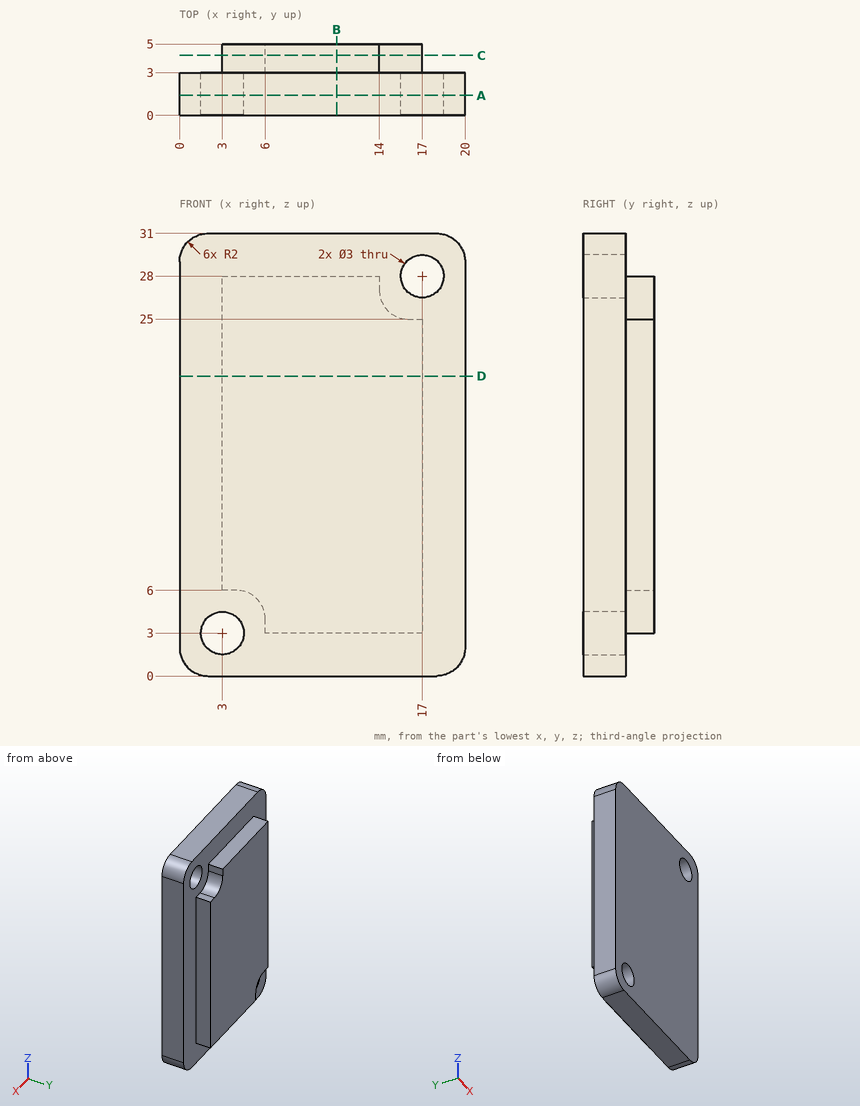
Print and shaded views of the part. All mm, measured from the part's lowest x, y and z. Round coordinates to 2 decimals unless told otherwise and drop trailing zeros. Order: outer loops, then holes, each group sorted by start corner. A loop starts at its lowest first (then second) coordinate and runs counter-clockwise, first axis right, second up.
Q1. Drop flat-ended pins along their axis: pin 1 (0.5 mm diameter, centred on x = 3.5, y = 3.5, fed in from -Z); pin 2 (3.5 mm diameter, centred on x = 17, z = 28, fed in from +Y); pin 3 (0.6 mm diameter, centred on x = 7.5, y = 4.5, fed in from +Z). Give the stop position or say it passes through.
Q2. Slice it at D-D (z = 21). Write the cut outline in (x, y), and give its area (3 significant figures).
Q3. Slice it at A-A (y = 1.4). Write the cut outline in (x, z).
Q4. Wall check: L1, parallel to X at y = 0.85, z = 28; L2, parallel to X at y = 1.3, z = 3; L3, parallel to Y at x = 1.75, z = 13.5. Give the ranges that are in metal, low to high.
Q5. Slice it at C-C (y = 4.2). Write the cut outline in (x, z).
Q6. Slice it at B-B (x = 11). Write the cut outline in (y, z), and give its area (3 significant figures).
Results below:
1. pin 1: stops at z = 6
1. pin 2: stops at y = 3
1. pin 3: stops at z = 28
2. outline: (0, 0) - (20, 0) - (20, 3) - (17, 3) - (17, 5) - (3, 5) - (3, 3) - (0, 3) - close
2. area: 88.0 mm2
3. outline: (0, 2) arc R2 ccw to (2, 0) - (18, 0) arc R2 ccw to (20, 2) - (20, 29) arc R2 ccw to (18, 31) - (2, 31) arc R2 ccw to (0, 29) - close; hole circle Ø3 at (3, 3); hole circle Ø3 at (17, 28)
4. L1: x = 0 to 15.5, 18.5 to 20
4. L2: x = 0 to 1.5, 4.5 to 20
4. L3: y = 0 to 3
5. outline: (3, 6) - (4, 6) arc R2 cw to (6, 4) - (6, 3) - (17, 3) - (17, 25) - (16, 25) arc R2 cw to (14, 27) - (14, 28) - (3, 28) - close
6. outline: (0, 0) - (3, 0) - (3, 3) - (5, 3) - (5, 28) - (3, 28) - (3, 31) - (0, 31) - close
6. area: 143 mm2
